Input: part model. Units: mm. Frame: model coordinates. Face numbers are marked on the shaded views. A direction names the side the tool comes from. Coordinates: 2 decimals unless noted, no trailing zeros. Write each loop counter-clockwise with the first axis right and the second up, starting at its lowest first coordinate (ties: lowest second). Pieces come first, ordered by that corner, then holes. Notation, with made-up numbers: M -2,1 L 21,1 A32 ccw 21,28 Z; hole C 9,67 d10. An arc over 180 degrees is marked long. Write each question's results on one line, items separated by ' | '. Start each with the question number.
1. Ray query, probe 1 along Y at (x, z) = (0, 2); probe 2 along Y at (x, z) = (1.5, 5.15); probe 3 along X at (y, z) = (-1.25, 2.45). Return the intervals inside material, ascending.
2. Section query A-A, the plane x = 0. Output: boundary loops of the cut face in (y, z).
3. Section query B-B, the plane z = 4. Output: boundary loops of the cut face in (x, y).
4. Section query C-C, the plane y = 4. Output: boundary loops of the cut face in (x, z).
5. First-contact query: pin 1 (3 mm diameter, centred on y = 6.5, z = 4.5, fed in from -X); pin 2 (2 mm diameter, centred on x = -7.5, z = 1, fed in from -Y); pin 3 (1 mm diameter, centred on x = -8, z = 5, fed in from -Y); pin 4 (2 mm diameter, centred on x = -7, y = -0.5, fed in from -Z). Flat tips, straight axial feed; report the tip coordinate or a pass-through.
6. Set-up query: the marked faces 4 and 5. Return all of +Z, -Z, +X, -X, +Y, -Y with unobstructed straight access to the full face (end or side cutting, diameter ignored); none if empty.
7. Section query D-D, the plane x = 6.25. Output: boundary loops of the cut face in (y, z).
8. Pull-direction query (X, two-part tool) for the marked faces 1, 2 and 3; classes: +X half, -X half, draft (parallel to the pull), parting line (faces both ways), or undercut.
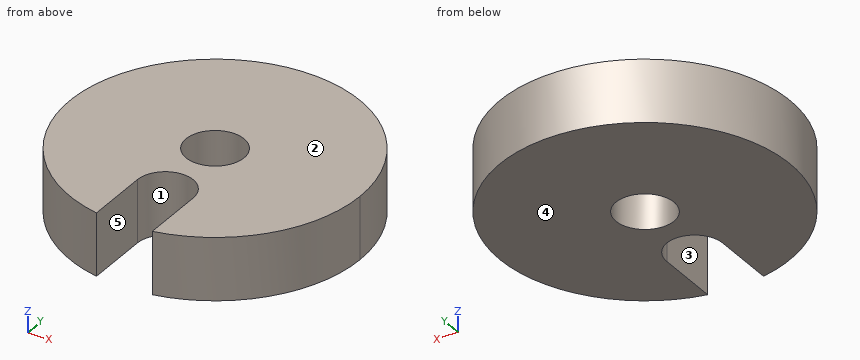
```python
from build123d import *

# Parameters (mm, degrees)
SZKIC1_R                    = 2.6
DODANIE_WYCI_GNI_CIE1_DEPTH = 5.6


with BuildPart() as part:
    # Szkic1 → Dodanie-wyciągnięcie1 (new body)
    with BuildSketch(Plane.XY):
        with BuildLine():
            Line((-2.5, -12.757350822), (-2.5, -7))
            ThreePointArc((-2.5, -7), (0, -4.5), (2.5, -7))
            Line((2.5, -7), (2.5, -12.757350822))
            ThreePointArc((2.5, -12.757350822), (10.03742995, -8.261355821), (13, 0))
            ThreePointArc((13, 0), (-8.261355821, 10.03742995), (-2.5, -12.757350822))
        make_face()
        Circle(SZKIC1_R, mode=Mode.SUBTRACT)
    extrude(amount=DODANIE_WYCI_GNI_CIE1_DEPTH)


solid = part.part
```
Answer:
1) probe 1: -4.5 to -2.6, 2.6 to 13 | probe 2: -5 to -2.12, 2.12 to 12.91 | probe 3: -12.94 to -2.28, 2.28 to 12.94
2) outline: M -4.5,0 L -2.6,0 L -2.6,5.6 L -4.5,5.6 Z; M 2.6,0 L 13,0 L 13,5.6 L 2.6,5.6 Z
3) outline: M -2.5,-12.76 L -2.5,-7 A2.5 cw 2.5,-7 L 2.5,-12.76 A13 ccw long Z; hole C 0,0 d5.2
4) outline: M -12.37,0 L 12.37,0 L 12.37,5.6 L -12.37,5.6 Z
5) pin 1: x = -12 | pin 2: y = -11.26 | pin 3: y = -10.62 | pin 4: z = 0
6) face 4: -Z, +X, -X, +Y, -Y | face 5: +Z, -Z, -Y
7) outline: M -11.4,0 L 11.4,0 L 11.4,5.6 L -11.4,5.6 Z
8) face 1: undercut | face 2: draft | face 3: undercut
